Check sheet for the modelled part. Datum: model origin and axes. Units: mm. Face numbers are marked on the shaded views. A direction names the side the tool comes from. Round coordinates to 2 decimals unless told otherwise and drop trailing zeros. Loops run counter-clockwise (first coordinate to the right, second up) from the corner with the lowest first, then second, coordinate; pieces in that order, holes last. Notation, with made-up numbers: (78.5, -25) -> (106.5, -25) arc R20 cw to (106.5, -3) -> close; hole circle Ø7 at (-17.5, 70). An arc over 180 degrees is marked (long way). Return JSON: item names as keys, results as strings.
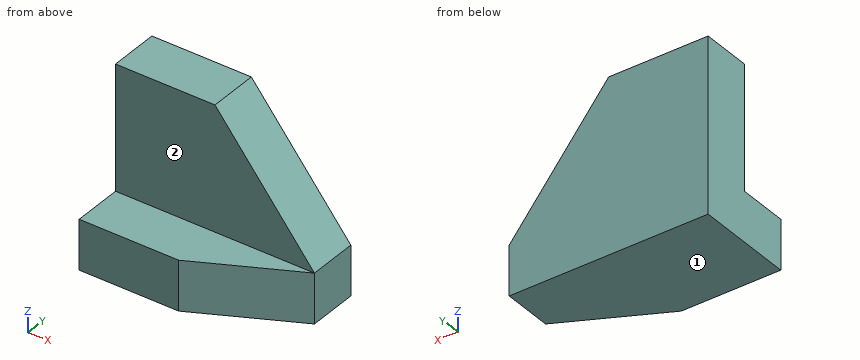
from build123d import *

# Parameters (mm, degrees)
F1_DEPTH = 12.7
F2_W     = 50.8
F2_H     = 12.7
F3_DEPTH = 12.7
F5_DEPTH = 25.4


with BuildPart() as f1:
    # F0 (on Front) → F1 (new body)
    with BuildSketch(Plane.XZ):
        Polygon((0, 44.45), (0, 0), (50.8, 0), (50.8, 12.7), (25.4, 44.45), align=None)
    extrude(amount=F1_DEPTH)

    # F2 (on face) → F3 (join)
    with BuildSketch(Plane.XZ.offset(12.7)):
        with Locations((25.4, 6.35)):
            Rectangle(F2_W, F2_H)
    extrude(amount=F3_DEPTH)

    # F4 (on face) → F5 (cut)
    with BuildSketch(Plane.XY.offset(12.7)):
        Polygon((50.8, -12.7), (25.4, -25.4), (50.8, -25.4), align=None)
    extrude(amount=-F5_DEPTH, mode=Mode.SUBTRACT)


solid = f1.part
Q1. Material ranges on line 1 (Y direction, x = 12, z = 37.5); line 2 (Z direction, x = 7.5, y = -16.5); line 3 (Z direction, x = 26.5, y = -1.5) (3 decimals), recorded low to high.
Results list:
{"line 1": "-12.7 to 0", "line 2": "0 to 12.7", "line 3": "0 to 43.075"}
Q2. Section check B-B (z = 8.5). Record the boundary of the cut face in (x, y), then the cut area to 3 significant figures.
Results list:
{"outline": "(0, -25.4) -> (25.4, -25.4) -> (50.8, -12.7) -> (50.8, 0) -> (0, 0) -> close", "area": "1,130 mm^2"}
Q3. Tool access check on the marked faces 1 and 2. Record the directions out of +Z, -Z, +X, -X, +Y, -Y that give a thin tool (end or side, any length) a straight path to the whole face; none if there is none.
Results list:
{"face 1": "-Z, +X, -X, +Y, -Y", "face 2": "+Z, +X, -X, -Y"}
Q4. Go/stop test with flat-tipped pins: pin 1 (8 mm diameter, centred on x = 13.5, z = 26, fed in from -Y); pin 2 (4 mm diameter, centred on x = 30.5, y = -16, fed in from +Z); pin 3 (8 mm diameter, centred on x = 31, y = -10, fed in from +Z). Record where each tip stops, or that it passes through.
Results list:
{"pin 1": "y = -12.7", "pin 2": "z = 12.7", "pin 3": "z = 42.45"}
Q5. Section check D-D (z = 34). Record the boundary of the cut face in (x, y), then the cut area to 3 significant figures.
Results list:
{"outline": "(0, -12.7) -> (33.76, -12.7) -> (33.76, 0) -> (0, 0) -> close", "area": "429 mm^2"}
Q6. Section check C-C (x = 15). Record the boundary of the cut face in (y, z), then the cut area to 3 significant figures.
Results list:
{"outline": "(-25.4, 0) -> (0, 0) -> (0, 44.45) -> (-12.7, 44.45) -> (-12.7, 12.7) -> (-25.4, 12.7) -> close", "area": "726 mm^2"}
Q7. Section check A-A (y = -1.75). Record the boundary of the cut face in (x, z).
Results list:
{"outline": "(0, 0) -> (50.8, 0) -> (50.8, 12.7) -> (25.4, 44.45) -> (0, 44.45) -> close"}
